Geometry: final body of the model. Coordinates: model frame, mm. Give positions to 0.01 mm unless a question says otherwise; leave off trailing zeros. Loops run counter-clockwise (first coordinate to the right, second up) from the corner with the lowest first, then second, coordinate; pieces in that order, holes last.
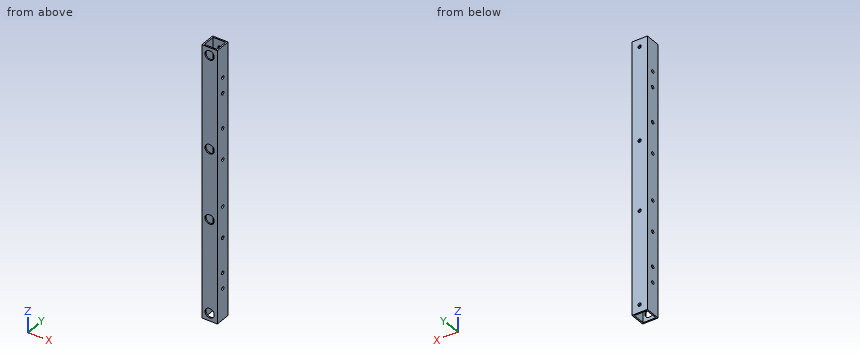
from build123d import *

# Parameters (mm, degrees)
SKETCH_3_W              = 20
SKETCH_3_H              = 20
SKETCH_3_W_2            = 16.4
SKETCH_3_H_2            = 16.4
EXTRUDE_1_DEPTH         = 350
HOLE_WIZARD_4_2_4_2_1_D = 4.2
HOLE_WIZARD_4_2_4_2_2_D = 4.2
CUT_EXTRUDE_2_REACH     = 353.141
SKETCH_11_R             = 6
HOLE_WIZARD_4_2_4_2_4_D = 4.2
HOLE_WIZARD_4_2_4_2_5_D = 4.2
CUT_EXTRUDE_3_REACH     = 353.141
SKETCH_16_R             = 6


with BuildPart() as part:
    # 草图3 → 凸台-拉伸1 (new body)
    with BuildSketch(Plane.XY):
        with Locations((10, 10)):
            Rectangle(SKETCH_3_W, SKETCH_3_H)
        with Locations((10, 10)):
            Rectangle(SKETCH_3_W_2, SKETCH_3_H_2, mode=Mode.SUBTRACT)
    extrude(amount=-EXTRUDE_1_DEPTH)

    # Ø4.2 (4.2) 直径孔1 (through all)
    with Locations(Plane(origin=(20, 10, -60), x_dir=(0, 1, 0), z_dir=(1, 0, 0))):
        with Locations((0, 0), (0, 20)):
            hole_wizard_4_2_4_2_1 = Hole(HOLE_WIZARD_4_2_4_2_1_D / 2)

    # 镜向1: Ø4.2 (4.2) 直径孔1 across plane
    add(hole_wizard_4_2_4_2_1.mirror(Plane.XY.offset(-175)), mode=Mode.SUBTRACT)

    # Ø4.2 (4.2) 直径孔2 (through all)
    with Locations(Plane(origin=(20, 10, -145), x_dir=(0, 1, 0), z_dir=(1, 0, 0))):
        with Locations((0, 0), (0, 40)):
            hole_wizard_4_2_4_2_2 = Hole(HOLE_WIZARD_4_2_4_2_2_D / 2)

    # 镜向2: Ø4.2 (4.2) 直径孔2 across plane
    add(hole_wizard_4_2_4_2_2.mirror(Plane.XY.offset(-175)), mode=Mode.SUBTRACT)

    # 草图11 → 切除-拉伸2 (cut, up to next)
    with BuildSketch(Plane.XZ, mode=Mode.PRIVATE) as cut_extrude_2_sk1:
        with Locations(Location((10, -10, 0), (0, 0, 270))):
            Circle(SKETCH_11_R)
    cut_extrude_2_tool1 = extrude(cut_extrude_2_sk1.sketch, amount=-CUT_EXTRUDE_2_REACH, mode=Mode.PRIVATE) & part.part
    # 草图11 → 切除-拉伸2 (cut, up to next)
    with BuildSketch(Plane.XZ, mode=Mode.PRIVATE) as cut_extrude_2_sk2:
        with Locations(Location((10, -340, 0), (0, 0, 270))):
            Circle(SKETCH_11_R)
    cut_extrude_2_tool2 = extrude(cut_extrude_2_sk2.sketch, amount=-CUT_EXTRUDE_2_REACH, mode=Mode.PRIVATE) & part.part
    add(cut_extrude_2_tool1.solids().sort_by_distance((10, 0, -10))[0], mode=Mode.SUBTRACT)
    add(cut_extrude_2_tool2.solids().sort_by_distance((10, 0, -340))[0], mode=Mode.SUBTRACT)

    # Ø4.2 (4.2) 直径孔4 (through all)
    with Locations(Plane(origin=(10, 20, -340), x_dir=(0, 0, 1), z_dir=(0, 1, 0))):
        with Locations((0, 0), (330, 0)):
            Hole(HOLE_WIZARD_4_2_4_2_4_D / 2)

    # Ø4.2 (4.2) 直径孔5 (through all)
    with Locations(Plane(origin=(10, 20, -220), x_dir=(0, 0, 1), z_dir=(0, 1, 0))):
        with Locations((0, 0), (90, 0)):
            Hole(HOLE_WIZARD_4_2_4_2_5_D / 2)

    # 草图16 → 切除-拉伸3 (cut, up to next)
    with BuildSketch(Plane.XZ, mode=Mode.PRIVATE) as cut_extrude_3_sk1:
        with Locations(Location((10, -130, 0), (0, 0, 270))):
            Circle(SKETCH_16_R)
    cut_extrude_3_tool1 = extrude(cut_extrude_3_sk1.sketch, amount=-CUT_EXTRUDE_3_REACH, mode=Mode.PRIVATE) & part.part
    # 草图16 → 切除-拉伸3 (cut, up to next)
    with BuildSketch(Plane.XZ, mode=Mode.PRIVATE) as cut_extrude_3_sk2:
        with Locations(Location((10, -220, 0), (0, 0, 270))):
            Circle(SKETCH_16_R)
    cut_extrude_3_tool2 = extrude(cut_extrude_3_sk2.sketch, amount=-CUT_EXTRUDE_3_REACH, mode=Mode.PRIVATE) & part.part
    add(cut_extrude_3_tool1.solids().sort_by_distance((10, 0, -130))[0], mode=Mode.SUBTRACT)
    add(cut_extrude_3_tool2.solids().sort_by_distance((10, 0, -220))[0], mode=Mode.SUBTRACT)


solid = part.part
Item 1: Ray query, probe 1 along Y at (x, z) = (18.8, -310); probe 2 along X at (y, z) = (14, -30). Return the intervals inside material, ascending.
Values follow:
probe 1: y = 0 to 7.9, 12.1 to 20
probe 2: x = 0 to 1.8, 18.2 to 20
Item 2: Pin query (flat end, axial travel): pin 1 (3.5 mm diameter, centred on y = 10, z = -145, fed in from +X); pin 2 (11 mm diameter, centred on x = 10, z = -340, fed in from -Y). Return the tip coordinate at first contact, or that it passes through.
Values follow:
pin 1: passes through
pin 2: stops at y = 18.2
Item 3: Section query A-A on y = 15. Return loops of the section in (x, z).
Values follow:
outline: (0, -350) - (1.8, -350) - (1.8, 0) - (0, 0) - close; (18.2, -350) - (20, -350) - (20, 0) - (18.2, 0) - close
Item 4: Section query B-B on z = -279. Return loops of the section in (x, y), plus the area to 3 significant figures.
Values follow:
outline: (0, 0) - (20, 0) - (20, 20) - (0, 20) - close; hole (1.8, 1.8) - (18.2, 1.8) - (18.2, 18.2) - (1.8, 18.2) - close
area: 131 mm2
